```python
from build123d import *

# Parameters (mm, degrees)
SKETCH1_W           = 100
SKETCH1_H           = 30
BOSS_EXTRUDE1_DEPTH = 1.5
SKETCH2_W           = 80
SKETCH2_H           = 15
SKETCH2_W_2         = 77
SKETCH2_H_2         = 12
EXTRUDE_THIN1_DEPTH = 10
SKETCH3_R           = 5
BOSS_EXTRUDE2_DEPTH = 10
SKETCH4_R           = 1.5
CUT_EXTRUDE1_DEPTH  = 10
FILLET1_R           = 5


with BuildPart() as part:
    # Sketch1 → Boss-Extrude1 (new body)
    with BuildSketch(Plane.XY):
        Rectangle(SKETCH1_W, SKETCH1_H)
    extrude(amount=BOSS_EXTRUDE1_DEPTH)

    # Sketch2 → Extrude-Thin1 (add)
    with BuildSketch(Plane.XY.offset(1.5)):
        Rectangle(SKETCH2_W, SKETCH2_H)
        Rectangle(SKETCH2_W_2, SKETCH2_H_2, mode=Mode.SUBTRACT)
    extrude(amount=EXTRUDE_THIN1_DEPTH)

    # Sketch3 → Boss-Extrude2 (add)
    with BuildSketch(Plane.XY.offset(1.5)):
        with Locations((-35, 0)):
            Circle(SKETCH3_R)
        with Locations((35, 0)):
            Circle(SKETCH3_R)
    extrude(amount=BOSS_EXTRUDE2_DEPTH)

    # Sketch4 → Cut-Extrude1 (cut)
    with BuildSketch(Plane.XY.offset(11.5)):
        with Locations((-35, 0)):
            Circle(SKETCH4_R)
        with Locations(Location((35, 0, 0), (0, 0, 180))):
            Circle(SKETCH4_R)
    extrude(amount=-CUT_EXTRUDE1_DEPTH, mode=Mode.SUBTRACT)

    # Fillet1
    # the kernel refuses this fillet: 5 mm, written as the material it adds along each edge
    with BuildSketch(Plane(origin=(38.5, -6, 1.5), x_dir=(0, 1, 0), z_dir=(0, 0, 1))) as fillet1_piece_1:
        with BuildLine():
            CenterArc((5, 4.288522873), FILLET1_R, 180, 59.059821395)
            Line((0, 4.288522873), (0, 0))
            Line((0, 0), (2.429285786, 0))
        make_face()
    extrude(amount=10)
    with BuildSketch(Plane(origin=(38.5, 6, 1.5), x_dir=(0, -1, 0), z_dir=(0, 0, 1))) as fillet1_piece_2:
        with BuildLine():
            CenterArc((5, -4.288522873), FILLET1_R, 120.940178605, 59.059821395)
            Line((0, -4.288522873), (0, 0))
            Line((0, 0), (2.429285786, 0))
        make_face()
    extrude(amount=10)
    with BuildSketch(Plane(origin=(-38.5, -6, 1.5), x_dir=(1, 0, 0), z_dir=(0, 0, 1))) as fillet1_piece_3:
        with BuildLine():
            CenterArc((4.288522873, 5), FILLET1_R, 210.940178605, 59.059821395)
            Line((0, 2.429285786), (0, 0))
            Line((0, 0), (4.288522873, 0))
        make_face()
    extrude(amount=10)
    with BuildSketch(Plane(origin=(-38.5, 6, 1.5), x_dir=(1, 0, 0), z_dir=(0, 0, 1))) as fillet1_piece_4:
        with BuildLine():
            CenterArc((4.288522873, -5), FILLET1_R, 90, 59.059821395)
            Line((0, -2.429285786), (0, 0))
            Line((0, 0), (4.288522873, 0))
        make_face()
    extrude(amount=10)
    # the kernel refuses this fillet: 5 mm, written as the material it takes off along each edge
    with BuildSketch(Plane(origin=(40, 7.5, 1.5), x_dir=(0, -1, 0), z_dir=(0, 0, 1)), Plane(origin=(40, -7.5, 1.5), x_dir=(-1, 0, 0), z_dir=(0, 0, 1)), Plane(origin=(-40, 7.5, 1.5), x_dir=(1, 0, 0), z_dir=(0, 0, 1))) as fillet1_2_piece_1:
        with BuildLine():
            CenterArc((FILLET1_R, -FILLET1_R), FILLET1_R, 90, 90)
            Line((0, -FILLET1_R), (0, 0))
            Line((0, 0), (FILLET1_R, 0))
        make_face()
    extrude(amount=22.5, mode=Mode.SUBTRACT)
    with BuildSketch(Plane(origin=(-40, -7.5, 1.5), x_dir=(1, 0, 0), z_dir=(0, 0, 1))) as fillet1_2_piece_2:
        with BuildLine():
            CenterArc((FILLET1_R, FILLET1_R), FILLET1_R, 180, 90)
            Line((0, FILLET1_R), (0, 0))
            Line((0, 0), (FILLET1_R, 0))
        make_face()
    extrude(amount=22.5, mode=Mode.SUBTRACT)
    with BuildSketch(Plane(origin=(-50, 15, -12.5), x_dir=(1, 0, 0), z_dir=(0, 0, 1)), Plane(origin=(-50, -15, -12.5), x_dir=(0, 1, 0), z_dir=(0, 0, 1))) as fillet1_2_piece_3:
        with BuildLine():
            CenterArc((FILLET1_R, -FILLET1_R), FILLET1_R, 90, 90)
            Line((0, -FILLET1_R), (0, 0))
            Line((0, 0), (FILLET1_R, 0))
        make_face()
    extrude(amount=26.5, mode=Mode.SUBTRACT)
    with BuildSketch(Plane(origin=(50, -15, -12.5), x_dir=(0, 1, 0), z_dir=(0, 0, 1)), Plane(origin=(50, 15, -12.5), x_dir=(-1, 0, 0), z_dir=(0, 0, 1))) as fillet1_2_piece_4:
        with BuildLine():
            CenterArc((FILLET1_R, FILLET1_R), FILLET1_R, 180, 90)
            Line((0, FILLET1_R), (0, 0))
            Line((0, 0), (FILLET1_R, 0))
        make_face()
    extrude(amount=26.5, mode=Mode.SUBTRACT)


solid = part.part
```
For this review, take the finished solid that the model builds, in its own axes (mm). A direction names the side the tool comes from. Give positions to 0.01 mm unless a question says otherwise; leave off trailing zeros. Write each loop counter-clockwise with the first axis right and the second up, starting at its lowest first coordinate (ties: lowest second). Pieces come first, ordered by that corner, then holes. Notation, with made-up numbers: M -27,17.5 L -5,17.5 A17 cw -5,37.5 Z; hole C 55.5,0.25 d3. An arc over 180 degrees is marked long. Answer as a JSON object with one key per item and string values. Group by question number.
Item 1: For probe 1 along Y at (x, z) = (-3, 10.5); probe 2 along Y at (x, z) = (35, 8); probe 3 along Z at (x, y) = (-7, 0.5), list the stretches that pass through material, from the lowest coordinate up. Write a range as [from, to].
Item 2: Consider section B-B on y = 0. Write out the cut boundary in (x, z), plus the area to 3 significant figures.
Item 3: Tool access review of faces 5 (the cylindrical face through (-48, 14, 1)), 6 (the flat face through (-35, 0, 1.5)), 7 (the flat face through (0, 7.5, 6)), 8 (the cylindrical face through (-38.5, 6.07, 6.43)): name each direction out of +Z, -Z, +X, -X, +Y, -Y from which nothing blocks a thin tool from reaching the whole face with its end or side.
Item 4: For pin 1 Ø3 at (x, z) = (-6, 8) entering from +Y; pin 2 Ø1.5 at (x, y) = (-35, 0) entering from +Z; pin 3 Ø1.5 at (y, z) = (1, 7) entering from +X, all flat-tipped, find the tip position at first contact; note any pin that passes through.
Item 5: Consider section C-C on x = 14.5. Write out the cut boundary in (y, z).
Item 6: Draft analysis for pull direction Y (two halves, no side actions). For faces 1 (the cylindrical face through (30, 0, 6)), 2 (the flat face through (-1, 0, 0)), 3 (the cylindrical face through (49, 13, 1)), 4 (the cylindrical face through (38.5, -6.07, 6.43)), state which applies: +Y half, -Y half, draft (parallel to the pull), parting line (faces both ways), or undercut.
Item 7: Consider section D-D on y = -9. Write out the cut boundary in (x, z).
Item 8: Consider section A-A on z = 6.75. Write out the cut boundary in (x, y), plus the area to 3 significant figures.
Check result:
{
 "1": {"probe 1": "y = [-7.5, -6], [6, 7.5]", "probe 2": "y = [-7.5, -5.94], [-5, -1.5], [1.5, 5], [5.94, 7.5]", "probe 3": "z = [0, 1.5]"},
 "2": {"outline": "M -50,0 L 50,0 L 50,1.5 L 40,1.5 L 40,11.5 L 36.5,11.5 L 36.5,1.5 L 33.5,1.5 L 33.5,11.5 L 30,11.5 L 30,1.5 L -30,1.5 L -30,11.5 L -33.5,11.5 L -33.5,1.5 L -36.5,1.5 L -36.5,11.5 L -40,11.5 L -40,1.5 L -50,1.5 Z", "area": "290 mm^2"},
 "3": {"face 5": "+Z, -Z, -X, +Y", "face 6": "+Z", "face 7": "+Z, +X, -X, +Y", "face 8": "+Z, -X, +Y"},
 "4": {"pin 1": "stops at y = 7.5", "pin 2": "stops at z = 1.5", "pin 3": "stops at x = 40"},
 "5": {"outline": "M -15,0 L 15,0 L 15,1.5 L 7.5,1.5 L 7.5,11.5 L 6,11.5 L 6,1.5 L -6,1.5 L -6,11.5 L -7.5,11.5 L -7.5,1.5 L -15,1.5 Z"},
 "6": {"face 1": "undercut", "face 2": "draft", "face 3": "+Y half", "face 4": "-Y half"},
 "7": {"outline": "M -50,0 L 50,0 L 50,1.5 L -50,1.5 Z"},
 "8": {"outline": "M -40,-2.5 A5 ccw -35,-7.5 L 35,-7.5 A5 ccw 40,-2.5 L 40,2.5 A5 ccw 35,7.5 L -35,7.5 A5 ccw -40,2.5 Z; hole M -38.5,-3.57 A5 ccw -34.21,-6 L 34.21,-6 A5 ccw 38.5,-3.57 A5 cw long 38.5,3.57 A5 ccw 34.21,6 L -34.21,6 A5 ccw -38.5,3.57 A5 cw long Z; hole C -35,0 d3; hole C 35,0 d3", "area": "395 mm^2"}
}
